```python
from build123d import *

# Parameters (mm, degrees)
F0_R     = 128.8146505864
F1_DEPTH = 25.4
F3_R     = 49.0141215923
F4_DEPTH = 50.8


# Not quite as in the source:
# - the program builds the solid bodies; features that only make, move or delete a surface that nothing else refers to are left out


with BuildPart() as f1:
    # F0 (on Front) → F1 (new body)
    with BuildSketch(Plane.XZ):
        with Locations((10.3380498641, 23.791786507)):
            Circle(F0_R)
        with BuildLine():
            ThreePointArc((48.5750728322, 28.0582736708), (55.5999914747, 14.8036448721), (58.026257129, 0))
            ThreePointArc((58.026257129, 0), (42.1859059552, -34.9036707218), (5.4861297438, -45.9630279004))
            ThreePointArc((5.4861297438, -45.9630279004), (-66.466433543, -36.001514495), (-48.743487455, 34.4420820545))
            ThreePointArc((-48.743487455, 34.4420820545), (0.9542816207, 81.3053730097), (48.7808239875, 32.5338840485))
            ThreePointArc((48.7808239875, 32.5338840485), (48.7293590503, 30.2937154281), (48.5750728322, 28.0582736708))
        make_face(mode=Mode.SUBTRACT)
    extrude(amount=F1_DEPTH)


with BuildPart() as f4:
    # F3 (on Front) → F4 (new body)
    with BuildSketch(Plane.XZ):
        Circle(F3_R)
    extrude(amount=F4_DEPTH)


solid = f4.part
```
For this review, take the finished solid that the model builds, in its own axes (mm). Round coordinates to 2 decimals unless told otherwise and drop trailing zeros. Loops run counter-clockwise (first coordinate to the right, second up) from the corner with the lowest first, then second, coordinate; pieces in that order, holes last.
Q1. To check wall thickness, follow line 1 along X through (y, z) = (-47.5, 21.5); line 2 along X through (y, z) = (-33, 17); line 3 along Z through (x, y) = (13.5, -30). State the ranges of each line that lie inside material, in increasing order.
Result sheet:
line 1: x = -44.05 to 44.05
line 2: x = -45.97 to 45.97
line 3: z = -47.12 to 47.12
Q2. Add section B-B on z = -39. Write out the cut boundary in (x, y), plus the area to 3 significant figures.
Result sheet:
outline: (-29.69, -50.8) - (29.69, -50.8) - (29.69, 0) - (-29.69, 0) - close
area: 3,020 mm2
Q3. Add section A-A on y = -37.5. Write out the cut boundary in (x, z), plus the area to 3 significant figures.
Result sheet:
outline: circle Ø98.03 at (0, 0)
area: 7,550 mm2
Q4. Insertion check: pin 1 Ø2 at (x, z) = (25, -24) entering from +Y; pin 2 Ø6 at (x, y) = (15.5, -26.5) entering from +Z; pin 3 Ø6 at (y, z) = (-6, 9) entering from -X; pin 4 Ø6 at (x, y) = (-1.5, -28.5) entering from -Z. Each pin has a flat end and moves straight along its axis. Give the tip position at first contact, or say it passes through.
Result sheet:
pin 1: stops at y = 0
pin 2: stops at z = 47.39
pin 3: stops at x = -48.65
pin 4: stops at z = -49.01
Q5. Add section C-C on x = 39. Write out the cut boundary in (y, z).
Result sheet:
outline: (-50.8, -29.69) - (0, -29.69) - (0, 29.69) - (-50.8, 29.69) - close
